Can you work these out from the model? Positions are in its coordinate system, mm. Give positions to 0.01 mm unless a question says otherwise; leave off trailing zeros. Write each loop counter-clockwise with the first axis right and the second up, starting at its lowest first coordinate (ties: lowest second). Pieces come first, ordered by that corner, then holes.
from build123d import *

# Parameters (mm, degrees)
SKETCH_1_W          = 300
SKETCH_1_H          = 200
EXTRUDE_1_DEPTH     = 5
SKETCH_2_R          = 1.75
SKETCH_2_W          = 30
SKETCH_2_H          = 80
CUT_EXTRUDE_1_DEPTH = 6


with BuildPart() as part:
    # ｽｹｯﾁ1 → ﾎﾞｽ - 押し出し1 (new body)
    with BuildSketch(Plane.XY):
        Rectangle(SKETCH_1_W, SKETCH_1_H)
    extrude(amount=EXTRUDE_1_DEPTH)

    # ｽｹｯﾁ2 → ｶｯﾄ - 押し出し1 (cut, through all)
    with BuildSketch(Plane.XY.offset(5)):
        with Locations((15, 30)):
            Circle(SKETCH_2_R)
        with Locations((-15, 30)):
            Circle(SKETCH_2_R)
        with Locations((-15, -30)):
            Circle(SKETCH_2_R)
        with Locations((15, -30)):
            Circle(SKETCH_2_R)
        with Locations((40, 0)):
            Rectangle(SKETCH_2_W, SKETCH_2_H)
        with Locations((-40, 0)):
            Rectangle(SKETCH_2_W, SKETCH_2_H)
    extrude(amount=-CUT_EXTRUDE_1_DEPTH, mode=Mode.SUBTRACT)


solid = part.part
(1) Imagine slicing it at B-B, the plane z = 3.5. Write out the boundary of the cut face in (x, y).
Returned:
outline: (-150, -100) - (150, -100) - (150, 100) - (-150, 100) - close; hole (-55, -40) - (-25, -40) - (-25, 40) - (-55, 40) - close; hole circle Ø3.5 at (-15, -30); hole circle Ø3.5 at (-15, 30); hole circle Ø3.5 at (15, -30); hole circle Ø3.5 at (15, 30); hole (25, -40) - (55, -40) - (55, 40) - (25, 40) - close
(2) If I drill on L1, parallel to X at y = 6, z = 1.25; L2, parallel to Y at x = 15, z = 2.6; L3, parallel to Y at x = -33, z = 4.7, over which ranges is the centre line in solid material (lowest first)?
Returned:
L1: x = -150 to -55, -25 to 25, 55 to 150
L2: y = -100 to -31.75, -28.25 to 28.25, 31.75 to 100
L3: y = -100 to -40, 40 to 100
(3) Will this pin go through, and if not, where does the flat tip stop? P1, Ø3, axis at x = 15, y = -30, coming from the -Z side.
Returned:
P1: passes through
(4) Imagine slicing it at C-C, the plane x = 34. Write out the boundary of the cut face in (y, z).
Returned:
outline: (-100, 0) - (-40, 0) - (-40, 5) - (-100, 5) - close; (40, 0) - (100, 0) - (100, 5) - (40, 5) - close
(5) Imagine slicing it at A-A, the plane y = 17. Write out the boundary of the cut face in (x, z), plus the area to 3 significant figures.
Returned:
outline: (-150, 0) - (-55, 0) - (-55, 5) - (-150, 5) - close; (-25, 0) - (25, 0) - (25, 5) - (-25, 5) - close; (55, 0) - (150, 0) - (150, 5) - (55, 5) - close
area: 1,200 mm2
